CAD build for the part. Positions are in the model's coordinates, mm. Face numbers are marked on the shaded views. A direction names the side the tool comes from. Coordinates: 2 decimals unless noted, no trailing zeros. Loops run counter-clockwise (first coordinate to the right, second up) from the corner with the lowest first, then second, coordinate; pieces in that order, holes last. Notation, with made-up numbers: (-10.75, -39.75) -> (39.25, -39.75) arc R21 cw to (39.25, -30.75) -> close; hole circle Ø10 at (53, 69). An arc over 180 degrees is marked (long way). Write each question's results on one line, items separated by ' | '.
from build123d import *

# Parameters (mm, degrees)
F1_DEPTH = 7
F0_R     = 0.7
F2_DEPTH = 3.5
F4_COUNT = 3


with BuildPart() as f1:
    # F0 (on Top) → F1 (new body)
    with BuildSketch(Plane.XY):
        with BuildLine():
            ThreePointArc((-12.382065884, 23.4666666667), (-7.2295689129, 18.0111162599), (0, 16))
            ThreePointArc((0, 16), (7.2295689129, 18.0111162599), (12.382065884, 23.4666666667))
            ThreePointArc((12.382065884, 23.4666666667), (13.5894981949, 26.6346562119), (14, 30))
            ThreePointArc((14, 30), (13.7458495795, 32.6554885307), (12.992625809, 35.2145637005))
            ThreePointArc((12.992625809, 35.2145637005), (-5.8818761492, 42.7044690155), (-12.382065884, 23.4666666667))
        make_face()
        with BuildLine():
            ThreePointArc((11, 30), (7.7781745931, 22.2218254069), (0, 19))
            ThreePointArc((0, 19), (-7.7781745931, 37.7781745931), (11, 30))
        make_face(mode=Mode.SUBTRACT)
        with BuildLine():
            ThreePointArc((5.1333333333, 9.7287660517), (9.4198372244, 5.6803755744), (11, 0))
            ThreePointArc((11, 0), (-7.7781745931, -7.7781745931), (0, 11))
            Line((0, 11), (0, 14))
            ThreePointArc((0, 14), (-6.8986101971, 12.1823305385), (-12.0058785253, 7.2013110498))
            ThreePointArc((-12.0058785253, 7.2013110498), (-3.7361544833, -13.4922625855), (14, 0))
            ThreePointArc((14, 0), (13.6478746634, 3.1201790289), (12.6092118325, 6.0834017591))
            ThreePointArc((12.6092118325, 6.0834017591), (12.3202312733, 6.649203063), (12.0058785253, 7.2013110498))
            ThreePointArc((12.0058785253, 7.2013110498), (9.6247415159, 10.166825992), (6.5333333333, 12.382065884))
            Line((6.5333333333, 12.382065884), (5.1333333333, 9.7287660517))
        make_face()
        with BuildLine():
            ThreePointArc((0, 11), (2.6441986906, 10.6774628674), (5.1333333333, 9.7287660517))
            Line((5.1333333333, 9.7287660517), (6.5333333333, 12.382065884))
            ThreePointArc((6.5333333333, 12.382065884), (3.3653437881, 13.5894981949), (0, 14))
            Line((0, 14), (0, 11))
        make_face()
        with BuildLine():
            ThreePointArc((0, 14), (3.3653437881, 13.5894981949), (6.5333333333, 12.382065884))
            Line((6.5333333333, 12.382065884), (7.6401623132, 14.4797438458))
            Line((7.6401623132, 14.4797438458), (12.382065884, 23.4666666667))
            ThreePointArc((12.382065884, 23.4666666667), (7.2295689129, 18.0111162599), (0, 16))
            Line((0, 16), (0, 14))
        make_face()
        with BuildLine():
            ThreePointArc((-12.0058785253, 7.2013110498), (-6.8986101971, 12.1823305385), (0, 14))
            Line((0, 14), (0, 16))
            ThreePointArc((0, 16), (-7.2295689129, 18.0111162599), (-12.382065884, 23.4666666667))
            Line((-12.382065884, 23.4666666667), (-8.9542338488, 16.9701908351))
            ThreePointArc((-8.9542338488, 16.9701908351), (-8.3782746662, 14.4999604986), (-9.0885864769, 12.0649606983))
            Line((-9.0885864769, 12.0649606983), (-12.0058785253, 7.2013110498))
        make_face()
        with BuildLine():
            ThreePointArc((14, 30), (13.5894981949, 26.6346562119), (12.382065884, 23.4666666667))
            Line((12.382065884, 23.4666666667), (15.8105643506, 29.9644055284))
            ThreePointArc((15.8105643506, 29.9644055284), (14.907806517, 30.8930023195), (14.2738299895, 32.0223107225))
            Line((14.2738299895, 32.0223107225), (12.992625809, 35.2145637005))
            ThreePointArc((12.992625809, 35.2145637005), (13.7458495795, 32.6554885307), (14, 30))
        make_face()
        with BuildLine():
            Line((7.6401623132, 14.4797438458), (6.5333333333, 12.382065884))
            ThreePointArc((6.5333333333, 12.382065884), (9.6247415159, 10.166825992), (12.0058785253, 7.2013110498))
            Line((12.0058785253, 7.2013110498), (7.6401623132, 14.4797438458))
        make_face()
    extrude(amount=F1_DEPTH)

    # F0 (on Top) → F2 (join)
    with BuildSketch(Plane.XY):
        with BuildLine():
            Line((7.6401623132, 14.4797438458), (12.0058785253, 7.2013110498))
            ThreePointArc((12.0058785253, 7.2013110498), (12.3202312733, 6.649203063), (12.6092118325, 6.0834017591))
            Line((12.6092118325, 6.0834017591), (20.7901645073, 21.588059159))
            ThreePointArc((20.7901645073, 21.588059159), (21.1448577828, 25.3984205095), (18.7013314535, 28.3435588795))
            Line((18.7013314535, 28.3435588795), (16.5807201594, 29.462488514))
            ThreePointArc((16.5807201594, 29.462488514), (16.1840828281, 29.6957099063), (15.8105643506, 29.9644055284))
            Line((15.8105643506, 29.9644055284), (12.382065884, 23.4666666667))
            Line((12.382065884, 23.4666666667), (7.6401623132, 14.4797438458))
        make_face()
        with Locations((15.9327194351, 20.1754820165)):
            Circle(F0_R, mode=Mode.SUBTRACT)
    extrude(amount=F2_DEPTH)

    # F4: F1 ×3 about axis
    f4_axis = Axis((0, 0, 10), (0, 0, 1))


with BuildPart() as f1_1:
    add(f1.part)
    for i in range(1, F4_COUNT):
        add(f1.part.rotate(f4_axis, i * 360 / F4_COUNT))


solid = f1_1.part
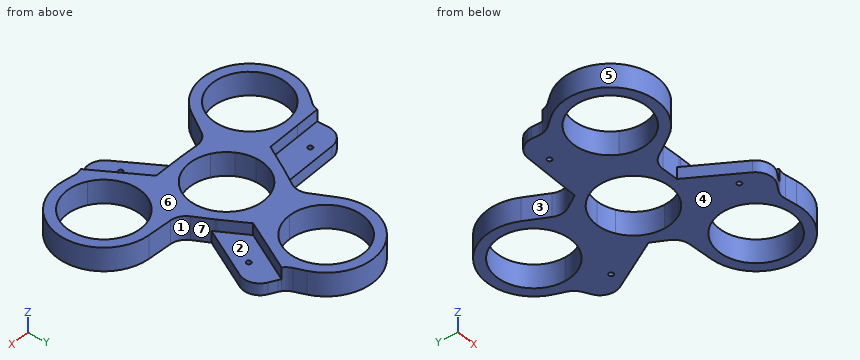
1) Drill centre lines: L1, parallel to Y at x = 0.5, z = 4; L2, parallel to X at y = -15, z = 5; L3, parallel to Y at x = 19.5, z = 2. Where is each one in solid material? Low to high. Write a range as from..to.
Outcome:
L1: y = -13.99..-10.99, 10.99..19.01, 40.99..43.99 | L2: x = -39.98..-36.98, -14.98..-9.11, 9.44..14.98, 36.98..39.98 | L3: y = -28.34..-23.89, -6.11..-0.74, 19.14..27.82
2) Two-plate mould, pull along Y, no slides. Class the marked faces 5, 6 and 7: pulls with the +Y half, pulls with the -Y half, needs draft (parallel to the pull), parting line crosses it, or undercut.
Outcome:
face 5: parting line crosses it | face 6: needs draft | face 7: undercut
3) Slice it at B-B (x = -17.5). Write the cut outline in (y, z), then the cut area to 3 significant figures.
Outcome:
outline: (-26.14, 0) -> (-22.01, 0) -> (-22.01, 7) -> (-26.14, 7) -> close; (-7.99, 0) -> (7.65, 0) -> (7.65, 3.5) -> (-0.67, 3.5) -> (-0.67, 7) -> (-7.99, 7) -> close | area: 109 mm^2
4) Slice it at D-D (z = 1). Count the separate pieces of the cut face and the enclosed holes in it, then the cut area to 3 significant figures.
Outcome:
separate pieces: 1 | enclosed holes: 7 | area: 1,670 mm^2
5) Slice it at C-C (x = -7). Write the cut outline in (y, z), then the cut area to 3 significant figures.
Outcome:
outline: (-14.01, 0) -> (-8.49, 0) -> (-8.49, 7) -> (-14.01, 7) -> close; (8.49, 0) -> (21.51, 0) -> (21.51, 7) -> (8.49, 7) -> close; (38.49, 0) -> (42.12, 0) -> (42.12, 7) -> (38.49, 7) -> close | area: 155 mm^2
6) Which spindle directions (+Z, -Z, +X, -X, +Y, -Y) get a long thin tool onto all of the face, cutting with end or side? Do the marked faces 1, 2, 3 and 4. Say none if no direction does.
Outcome:
face 1: +Z, -Z, +X | face 2: +Z, +X | face 3: +Z, -Z, -X | face 4: -Z, +X, -X, +Y, -Y
7) Pin check, flat tips, straight feed: pin 1 (12 mm diameter, centred on x = -4.5, y = -23, fed in from +Z); pin 2 (4.5 mm diameter, centred on x = -19, y = 2.5, fed in from +Z); pin 3 (2 mm diameter, centred on y = 5, z = 5, fed in from +X); pin 4 (3 mm diameter, centred on y = 13, z = 2, fed in from +X). Stop position of each tip, or through.
Outcome:
pin 1: passes through | pin 2: stops at z = 3.5 | pin 3: stops at x = 13.79 | pin 4: stops at x = 17.05
8) Slice it at A-A (y = -19). Write the cut outline in (x, z), then the cut area to 3 significant figures.
Outcome:
outline: (-39.4, 0) -> (-36.23, 0) -> (-36.23, 7) -> (-39.4, 7) -> close; (-15.73, 0) -> (-11.96, 0) -> (-11.96, 7) -> (-15.73, 7) -> close; (2.13, 0) -> (15.73, 0) -> (15.73, 7) -> (11.96, 7) -> (11.96, 3.5) -> (2.13, 3.5) -> close; (36.23, 0) -> (39.4, 0) -> (39.4, 7) -> (36.23, 7) -> close | area: 132 mm^2
